Read the model definition and answer for the solid it produces. Units are mm, in the model's axes. A direction names the side the tool comes from. Round coordinates to 2 decimals unless told otherwise and drop trailing zeros. Loops run counter-clockwise (first coordinate to the right, second up) from the corner with the lowest first, then second, coordinate; pieces in that order, holes last. Notation, with made-up numbers: M 9.5,8 L 51.5,8 A36 ccw 51.5,44 Z; hole C -11,-21 d8. An arc over 180 degrees is marked long. Answer as CSV lines item,"result".
```python
from build123d import *

# Parameters (mm, degrees)
SKETCH_1_W          = 80
SKETCH_1_H          = 56
EXTRUDE_1_DEPTH     = 200
CUT_EXTRUDE_1_DEPTH = 52
SKETCH_3_R          = 3.5
SKETCH_3_R_2        = 13
CUT_EXTRUDE_2_DEPTH = 10
SKETCH_5_R          = 8
SKETCH_5_R_2        = 3
CUT_EXTRUDE_4_DEPTH = 10
SKETCH_6_R          = 3.500000002
SKETCH_6_R_2        = 3.5
CUT_EXTRUDE_5_DEPTH = 10
SKETCH_7_W          = 90
SKETCH_7_H          = 40
CUT_EXTRUDE_6_DEPTH = 81


with BuildPart() as part:
    # 草图1 → 凸台-拉伸1 (new body)
    with BuildSketch(Plane.XY):
        Rectangle(SKETCH_1_W, SKETCH_1_H)
    extrude(amount=-EXTRUDE_1_DEPTH)

    # 草图2 → 切除-拉伸1 (cut)
    with BuildSketch(Plane(origin=(0, 28, 0), x_dir=(1, 0, 0), z_dir=(0, 1, 0))):
        with BuildLine():
            ThreePointArc((-36, 193), (-35.121320344, 195.121320344), (-33, 196))
            Line((-33, 196), (33, 196))
            ThreePointArc((33, 196), (35.121320344, 195.121320344), (36, 193))
            Line((36, 193), (36, 7))
            ThreePointArc((36, 7), (35.121320344, 4.878679656), (33, 4))
            Line((33, 4), (-33, 4))
            ThreePointArc((-33, 4), (-35.121320344, 4.878679656), (-36, 7))
            Line((-36, 7), (-36, 193))
        make_face()
    extrude(amount=-CUT_EXTRUDE_1_DEPTH, mode=Mode.SUBTRACT)

    # 草图3 → 切除-拉伸2 (cut)
    with BuildSketch(Plane.XY):
        with Locations((-28, 2)):
            Circle(SKETCH_3_R)
        with Locations((0, 2)):
            Circle(SKETCH_3_R_2)
        with Locations((28, 2)):
            Circle(SKETCH_3_R)
    extrude(amount=-CUT_EXTRUDE_2_DEPTH, mode=Mode.SUBTRACT)

    # 草图5 → 切除-拉伸4 (cut)
    with BuildSketch(Plane(origin=(0, 0, -200), x_dir=(-1, 0, 0), z_dir=(0, 0, -1))):
        with Locations((0, 2)):
            Circle(SKETCH_5_R)
        with Locations((25.5, 2)):
            Circle(SKETCH_5_R_2)
        with Locations((-25.5, 2)):
            Circle(SKETCH_5_R_2)
    extrude(amount=-CUT_EXTRUDE_4_DEPTH, mode=Mode.SUBTRACT)

    # 草图6 → 切除-拉伸5 (cut)
    with BuildSketch(Plane(origin=(0, -24, 0), x_dir=(1, 0, 0), z_dir=(0, 1, 0))):
        with Locations((-16, 166.5)):
            Circle(SKETCH_6_R)
        with Locations((-16, 113.5)):
            Circle(SKETCH_6_R_2)
    extrude(amount=-CUT_EXTRUDE_5_DEPTH, mode=Mode.SUBTRACT)

    # 草图7 → 切除-拉伸6 (cut, through all)
    with BuildSketch(Plane.ZY.offset(40)):
        with Locations((-113.014709347, 0)):
            Rectangle(SKETCH_7_W, SKETCH_7_H)
    extrude(amount=-CUT_EXTRUDE_6_DEPTH, mode=Mode.SUBTRACT)


solid = part.part
```
1) Find section A-A, the plane x = -16. Give the vertices of the cut face in (y, z), then the cut area to 3 significant figures.
Evaluation:
outline,"M -28,-200 L 28,-200 L 28,-196 L -24,-196 L -24,-170 L -28,-170 Z; M -28,-163 L -24,-163 L -24,-117 L -28,-117 Z; M -28,-110 L -24,-110 L -24,-4 L 28,-4 L 28,0 L -28,0 Z"
area,"1,160 mm^2"
2) Straight lines are drawn through the part: line 1 (Z direction, x = -16, y = -27.05); line 2 (X direction, y = 3.5, z = -30); line 3 (Z direction, x = 20, y = 16). For each, find the intervals that lie inside material, in ascending order.
Evaluation:
line 1,"z = -200 to -170, -163 to -117, -110 to 0"
line 2,"x = -40 to -36, 36 to 40"
line 3,"z = -200 to -196, -4 to 0"
3) Find section B-B, the plane z = -80. Give the vertices of the cut face in (x, y).
Evaluation:
outline,"M -40,-28 L 40,-28 L 40,-20 L 36,-20 L 36,-24 L -36,-24 L -36,-20 L -40,-20 Z; M -40,20 L -36,20 L -36,28 L -40,28 Z; M 36,20 L 40,20 L 40,28 L 36,28 Z"
4) Each of these flat-tipped pins is pushed along its axis until it touches: P1, Ø5.5, axis at x = -16, z = -166.5, coming from the -Y side; P2, Ø1.5, axis at y = 8, z = -157.5, coming from the +X side; P3, Ø6.5, axis at x = -28, y = 2, coming from the +Z side; P4, Ø9, axis at x = -16, z = -113.5, coming from the +Y side. Where does it stop, or does it pass through?
Evaluation:
P1,"passes through"
P2,"stops at x = 40"
P3,"stops at z = -196"
P4,"stops at y = -24"
5) Find section C-C, the plane z = -113.5. Give the vertices of the cut face in (x, y).
Evaluation:
outline,"M -40,-28 L -19.5,-28 L -19.5,-24 L -36,-24 L -36,-20 L -40,-20 Z; M -40,20 L -36,20 L -36,28 L -40,28 Z; M -12.5,-28 L 40,-28 L 40,-20 L 36,-20 L 36,-24 L -12.5,-24 Z; M 36,20 L 40,20 L 40,28 L 36,28 Z"
6) Find section D-D, the plane z = -166.5. Give the vertices of the cut face in (x, y).
Evaluation:
outline,"M -40,-28 L -19.5,-28 L -19.5,-24 L -36,-24 L -36,28 L -40,28 Z; M -12.5,-28 L 40,-28 L 40,28 L 36,28 L 36,-24 L -12.5,-24 Z"
7) Determine the mould class of faces 4 (the cylindrical face through (31.34, 3.05, -1.97)), 5 (the flat face through (38, 0, -68.015)), 6 (the flat face through (1, -24, -101)) for opening direction Z: released by +Z, released by -Z, zero draft, split by the parting line, or undercut.
Evaluation:
face 4,"zero draft"
face 5,"undercut"
face 6,"undercut"
8) A tool of negligible diameter and unlimited length cuts with its end or side. For faces 1 (the flat face through (7, 8, -196)), 2 (the cylindrical face through (28.5, 2.1, -198)), 3 (the flat face through (-38, 0, -158.015)), from which of +Z, -Z, +X, -X, +Y, -Y can it reach the whole face along a straight path? Write none if from no direction.
Evaluation:
face 1,"+Y"
face 2,"-Z"
face 3,"+X, -X"
